Input: part model. Units: mm. Frame: model coordinates. A direction names the side the tool comes from. Round coordinates to 2 decimals unless told otherwise and drop trailing zeros. Loops run counter-clockwise (first coordinate to the right, second up) from the corner with the lowest first, then second, coordinate; pieces in that order, holes last. Notation, with made-up numbers: M -10.5,88.5 L 21.5,88.5 A23 cw 21.5,100.5 Z; hole C 79,-12 d5. An arc over 180 degrees is marked long. Return JSON: item names as keys, results as strings. Group by question number.
1) Section C-C (x = -2.5). Output: boundary loops of the cut face in (y, z), plus the area to 3 significant figures.
2) Section B-B (y = 0.5). Count the separate pieces of the cut face and the enclosed holes in it, plus the area to 3 significant figures.
3) Access query for faces 1 (the face through (-13.1, 0.5, -2.7)), 2 (the face through (-12.336, 0.507, -23.515)). Directions: +Z, -Z, +X, -X, +Y, -Y. A direction counts if a zero-diameter tool reaches every point of the face in a straight line with its end or side. Return the directions, or none.
4) Section A-A (z = -31.5). Output: boundary loops of the cut face in (x, y), plus the area to 3 significant figures.
5) Contact query for a flat-ended pin moving along its axis: P1, Ø0.5, axis at x = -14.5, y = 0.5, coming from the +Z side. Output: stop coordinate, or through.
6) Mould query, pull axis X, two halves, no side actions, for faces 3 (the face through (11.782, 0.507, -19.395)), 4 (the face through (-14.8, 0.5, -6.5)), 5 (the face through (13.8, 0.5, -16.3)), 6 (the face through (-14.6, 0.5, -38)). Classes: +X half, -X half, draft (parallel to the pull), parting line (faces both ways), or undercut.
7) Material intervals for line 1 (X direction, y = 0.85, z = -18.8); line 2 (X direction, y = 0.2, z = -14); line 3 (Z direction, x = -2, y = 0.4), sorted ascending. Write a range as from..to.
from build123d import *

# Parameters (mm, degrees)
BOSS_EXTRU_1_DEPTH      = 1
ESQUISSE2_R             = 0.6
ENL_V_MAT_EXTRU_1_DEPTH = 1


with BuildPart() as part:
    # Esquisse1 → Boss.-Extru.1 (new body)
    with BuildSketch(Plane(origin=(0, 0, 0), x_dir=(1, 0, 0), z_dir=(0, 1, 0))):
        with BuildLine():
            Line((-13.1, 0), (-13.1, 5.5))
            ThreePointArc((-13.1, 5.5), (-13.392893219, 6.207106781), (-14.1, 6.5))
            Line((-14.1, 6.5), (-15.6, 6.5))
            Line((-15.6, 6.5), (-15.6, 37))
            Line((-15.6, 37), (-13.6, 39))
            Line((-13.6, 39), (13.6, 39))
            Line((13.6, 39), (15.6, 37))
            Line((15.6, 37), (15.6, 0))
            Line((15.6, 0), (4.8, 0))
            Line((4.8, 0), (4.8, 0.3))
            ThreePointArc((4.8, 0.3), (4.594974747, 0.794974747), (4.1, 1))
            Line((4.1, 1), (-4.1, 1))
            ThreePointArc((-4.1, 1), (-4.594974747, 0.794974747), (-4.8, 0.3))
            Line((-4.8, 0.3), (-4.8, 0))
            Line((-4.8, 0), (-13.1, 0))
        make_face()
    extrude(amount=BOSS_EXTRU_1_DEPTH)

    # Esquisse2 → Enlèv. mat.-Extru.1 (cut)
    with BuildSketch(Plane(origin=(0, 1, 0), x_dir=(1, 0, 0), z_dir=(0, 1, 0))):
        with Locations((14.4, 31.5)):
            Circle(ESQUISSE2_R)
        with Locations((11.86, 31.5)):
            Circle(ESQUISSE2_R)
        with Locations((11.86, 28.96)):
            Circle(ESQUISSE2_R)
        with Locations((11.86, 26.42)):
            Circle(ESQUISSE2_R)
        with Locations((11.86, 23.88)):
            Circle(ESQUISSE2_R)
        with Locations((11.86, 21.34)):
            Circle(ESQUISSE2_R)
        with Locations((11.86, 18.8)):
            Circle(ESQUISSE2_R)
        with Locations((11.86, 16.26)):
            Circle(ESQUISSE2_R)
        with Locations((11.86, 13.72)):
            Circle(ESQUISSE2_R)
        with Locations((11.86, 11.18)):
            Circle(ESQUISSE2_R)
        with Locations((11.86, 8.64)):
            Circle(ESQUISSE2_R)
        with Locations((14.4, 28.96)):
            Circle(ESQUISSE2_R)
        with Locations((14.4, 26.42)):
            Circle(ESQUISSE2_R)
        with Locations((14.4, 23.88)):
            Circle(ESQUISSE2_R)
        with Locations((14.4, 21.34)):
            Circle(ESQUISSE2_R)
        with Locations((14.4, 18.8)):
            Circle(ESQUISSE2_R)
        with Locations((14.4, 16.26)):
            Circle(ESQUISSE2_R)
        with Locations((14.4, 13.72)):
            Circle(ESQUISSE2_R)
        with Locations((14.4, 11.18)):
            Circle(ESQUISSE2_R)
        with Locations((14.4, 8.64)):
            Circle(ESQUISSE2_R)
        with Locations((-14.4, 8.64)):
            Circle(ESQUISSE2_R)
        with Locations((-14.4, 11.18)):
            Circle(ESQUISSE2_R)
        with Locations((-14.4, 13.72)):
            Circle(ESQUISSE2_R)
        with Locations((-14.4, 16.26)):
            Circle(ESQUISSE2_R)
        with Locations((-14.4, 18.8)):
            Circle(ESQUISSE2_R)
        with Locations((-14.4, 21.34)):
            Circle(ESQUISSE2_R)
        with Locations((-14.4, 23.88)):
            Circle(ESQUISSE2_R)
        with Locations((-14.4, 26.42)):
            Circle(ESQUISSE2_R)
        with Locations((-14.4, 28.96)):
            Circle(ESQUISSE2_R)
        with Locations((-11.86, 8.64)):
            Circle(ESQUISSE2_R)
        with Locations((-11.86, 11.18)):
            Circle(ESQUISSE2_R)
        with Locations((-11.86, 13.72)):
            Circle(ESQUISSE2_R)
        with Locations((-11.86, 16.26)):
            Circle(ESQUISSE2_R)
        with Locations((-11.86, 18.8)):
            Circle(ESQUISSE2_R)
        with Locations((-11.86, 21.34)):
            Circle(ESQUISSE2_R)
        with Locations((-11.86, 23.88)):
            Circle(ESQUISSE2_R)
        with Locations((-11.86, 26.42)):
            Circle(ESQUISSE2_R)
        with Locations((-11.86, 28.96)):
            Circle(ESQUISSE2_R)
        with Locations((-11.86, 31.5)):
            Circle(ESQUISSE2_R)
        with Locations((-14.4, 31.5)):
            Circle(ESQUISSE2_R)
    extrude(amount=-ENL_V_MAT_EXTRU_1_DEPTH, mode=Mode.SUBTRACT)


solid = part.part
Returned:
{
 "1": {"outline": "M 0,-39 L 1,-39 L 1,-1 L 0,-1 Z", "area": "38.0 mm^2"},
 "2": {"separate pieces": "1", "enclosed holes": "40", "area": "1,140 mm^2"},
 "3": {"face 1": "+Z, -X, +Y, -Y", "face 2": "+Y, -Y"},
 "4": {"outline": "M -15.6,0 L -15,0 L -15,1 L -15.6,1 Z; M -13.8,0 L -12.46,0 L -12.46,1 L -13.8,1 Z; M -11.26,0 L 11.26,0 L 11.26,1 L -11.26,1 Z; M 12.46,0 L 13.8,0 L 13.8,1 L 12.46,1 Z; M 15,0 L 15.6,0 L 15.6,1 L 15,1 Z", "area": "26.4 mm^2"},
 "5": {"P1": "stops at z = -6.5"},
 "6": {"face 3": "undercut", "face 4": "draft", "face 5": "undercut", "face 6": "-X half"},
 "7": {"line 1": "x = -15.6..-15, -13.8..-12.46, -11.26..11.26, 12.46..13.8, 15..15.6", "line 2": "x = -15.6..-14.93, -13.87..-12.39, -11.33..11.33, 12.39..13.87, 14.93..15.6", "line 3": "z = -39..-1"}
}
